```python
from build123d import *

# Parameters (mm, degrees)
F1_DEPTH = 3.5
F2_DEPTH = 1.5
F4_DEPTH = 3.5


with BuildPart() as f1:
    # F0 (on Right) → F1 (new body, symmetric)
    with BuildSketch(Plane.YZ):
        with BuildLine():
            ThreePointArc((-16, 0), (0, -16), (16, 0))
            Line((16, 0), (14.5, 0))
            ThreePointArc((14.5, 0), (0, -14.5), (-14.5, 0))
            Line((-14.5, 0), (-16, 0))
        make_face()
        with BuildLine():
            Line((18, 0), (16, 0))
            ThreePointArc((16, 0), (0, -16), (-16, 0))
            Line((-16, 0), (-18, 0))
            ThreePointArc((-18, 0), (0, -18), (18, 0))
        make_face()
    extrude(amount=F1_DEPTH, both=True)

    # F0 (on Right) → F2 (cut, symmetric)
    with BuildSketch(Plane.YZ):
        with BuildLine():
            ThreePointArc((-16, 0), (0, -16), (16, 0))
            Line((16, 0), (14.5, 0))
            ThreePointArc((14.5, 0), (0, -14.5), (-14.5, 0))
            Line((-14.5, 0), (-16, 0))
        make_face()
    extrude(amount=F2_DEPTH, both=True, mode=Mode.SUBTRACT)

    # F3 (on Right) → F4 (join, symmetric)
    with BuildSketch(Plane.YZ):
        Polygon((8, -32.6522623003), (-8, -32.6522623003), (-10, -32.6522623003), (-15, -32.6522623003), (-15, -35.1522623003), (-3, -35.1522623003), (3, -35.1522623003), (15, -35.1522623003), (15, -32.6522623003), (10, -32.6522623003), align=None)
        with BuildLine():
            Line((3, -15.1522623003), (-3, -15.1522623003))
            Line((-3, -15.1522623003), (-3, -27.6522623003))
            ThreePointArc((-3, -27.6522623003), (-4.4644660941, -31.1877962062), (-8, -32.6522623003))
            Line((-8, -32.6522623003), (8, -32.6522623003))
            ThreePointArc((8, -32.6522623003), (4.4644660941, -31.1877962062), (3, -27.6522623003))
            Line((3, -27.6522623003), (3, -15.1522623003))
        make_face()
    extrude(amount=F4_DEPTH, both=True)


solid = f1.part
```
The model under review builds one solid part; all positions refer to its coordinate system, in mm. A direction names the side the tool comes from. Round coordinates to 2 decimals unless told otherwise and drop trailing zeros. Order: outer loops, then holes, each group sorted by start corner. A loop starts at its lowest first (then second) coordinate and runs counter-clockwise, first axis right, second up. Notation, with made-up numbers: M 51,4.5 L 107,4.5 A34 cw 107,35.5 Z; hole C -32,13.5 d10. An arc over 180 degrees is marked long. Use a Markdown table: item, result.
1) Insertion check: pin 1 (2 mm diameter, centred on x = 0, y = 13, fed in from +Z); pin 2 (3 mm diameter, centred on x = 0.5, y = 8, fed in from +Z); pin 3 (2 mm diameter, centred on x = -1.5, z = -34.5, fed in from +Y). Each pin has a flat end and moves straight along its axis. Give the tip position at first contact, or say it passes through.
Report:
| item | result |
|---|---|
| pin 1 | z = -7.75 |
| pin 2 | z = -11.27 |
| pin 3 | y = 15 |
2) Consider section B-B (y = 0). Write out the cut boundary in (x, z).
Report:
| item | result |
|---|---|
| outline | M -3.5,-35.15 L 3.5,-35.15 L 3.5,-14.5 L 1.5,-14.5 L 1.5,-15.15 L -1.5,-15.15 L -1.5,-14.5 L -3.5,-14.5 Z |
3) Draft analysis for pull direction Z (two halves, no side actions). For faces 1 (the face through (0, 15, -34)), 2 (the face through (0, -11, -32.652)), 3 (the face through (0.021, -12.427, -10.078)), state which applies: released by +Z, released by -Z, zero draft, split by the parting line, or undercut.
Report:
| item | result |
|---|---|
| face 1 | zero draft |
| face 2 | undercut |
| face 3 | released by +Z |
4) Consider section A-A (x = 2.5). Write out the cut boundary in (y, z).
Report:
| item | result |
|---|---|
| outline | M -18,0 A18 ccw -3,-17.75 L -3,-27.65 A5 cw -8,-32.65 L -15,-32.65 L -15,-35.15 L 15,-35.15 L 15,-32.65 L 8,-32.65 A5 cw 3,-27.65 L 3,-17.75 A18 ccw 18,0 L 14.5,0 A14.5 cw -14.5,0 Z |
5) Consider section D-D (z = -6). Write out the cut boundary in (x, y), then the cut area to 3 significant figures.
Report:
| item | result |
|---|---|
| outline | M -3.5,-16.97 L 3.5,-16.97 L 3.5,-13.2 L 1.5,-13.2 L 1.5,-14.83 L -1.5,-14.83 L -1.5,-13.2 L -3.5,-13.2 Z; M -3.5,13.2 L -1.5,13.2 L -1.5,14.83 L 1.5,14.83 L 1.5,13.2 L 3.5,13.2 L 3.5,16.97 L -3.5,16.97 Z |
| area | 43.0 mm^2 |
6) Tool access review of faces 4 (the face through (0, 3, -23)), 5 (the face through (0.049, -13.861, -11.483)), 6 (the face through (1.5, -1, -15)): name each direction out of +Z, -Z, +X, -X, +Y, -Y from which nothing blocks a thin tool from reaching the whole face with its end or side.
Report:
| item | result |
|---|---|
| face 4 | +X, -X, +Y |
| face 5 | +X, -X, -Y |
| face 6 | +Z |
7) Wall thickness on line 1 along X through (y, z) = (-14.5, -2); line 2 along Y through (x, z) = (-0.5, -3.5); line 3 along Y through (x, z) = (-0.5, -21.5): over which ranges is each line inside the solid? List them lowest first. Write a range as [from, to].
Report:
| item | result |
|---|---|
| line 1 | [-3.5, -1.5], [1.5, 3.5] |
| line 2 | [-17.66, -15.61], [15.61, 17.66] |
| line 3 | [-3, 3] |
8) Consider section C-C (y = -13). Write out the cut boundary in (x, z).
Report:
| item | result |
|---|---|
| outline | M -3.5,-35.15 L 3.5,-35.15 L 3.5,-32.65 L -3.5,-32.65 Z; M -3.5,-12.45 L 3.5,-12.45 L 3.5,-6.42 L 1.5,-6.42 L 1.5,-9.33 L -1.5,-9.33 L -1.5,-6.42 L -3.5,-6.42 Z |
